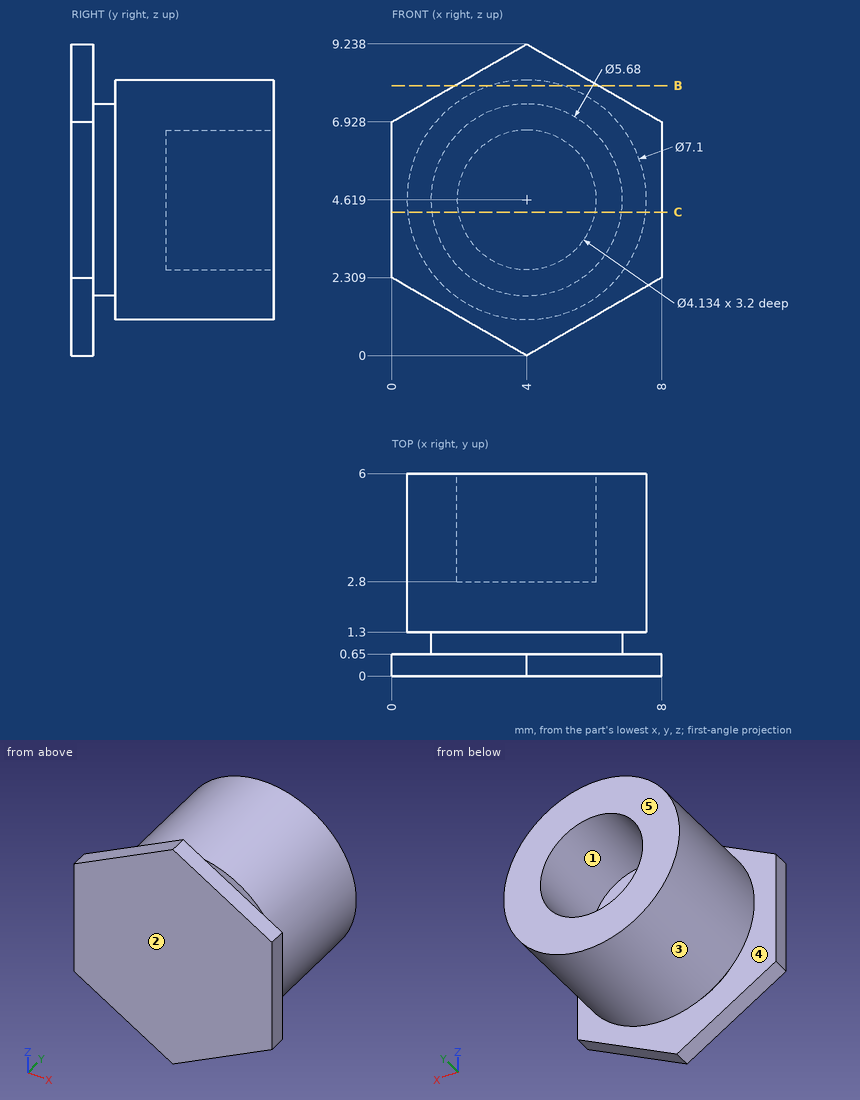
Part print with two shaded views. Sizes in mm from the minimum x, y, z corner. A direction names the side the tool comes from. Coordinates: 2 decimals unless noted, no trailing zeros. Write each loop counter-clockwise with the first axis right and the second up, starting at its lowest first coordinate (ties: lowest second). Pieces come first, ordered by that corner, then holes.
(1) Mould opens along Z. For the marked faces 1, 2 and 3 say: pulls with the +Z half, pulls with the -Z half, needs draft (parallel to the pull), parting line crosses it, or undercut.
(2) Cut at C-C on z = 4.25. List the corners of the cut face in (x, y).
(3) 3-axis set-ups, long thin cutter, end or side, ignore diameter. For the marked faces 4 and 5: which of +Z, -Z, +X, -X, +Y, -Y reach the whole face in a straight line?
(4) Cut at B-B on z = 8. List the corners of the cut face in (x, y).
(5) Pin check, flat tips, straight feed: pin 1 Ø2 at (x, z) = (3.5, 5) entering from +Y; pin 2 Ø3 at (x, y) = (6, 1) entering from +Z (1 decimal). Stop position of each tip, or through.
(6) Drill centre lines: line 1 (Z direction, x = 4, y = 4.1) (1 decimal); line 2 (Y direction, x = 3, z = 6); line 3 (Z direction, x = 2.75, y = 4.25) (1 decimal). Where is each one in solid material? Low to high.
Working result:
1. face 1: undercut
1. face 2: needs draft
1. face 3: parting line crosses it
2. outline: (0, 0) - (8, 0) - (8, 0.65) - (6.82, 0.65) - (6.82, 1.3) - (7.53, 1.3) - (7.53, 6) - (6.03, 6) - (6.03, 2.8) - (1.97, 2.8) - (1.97, 6) - (0.47, 6) - (0.47, 1.3) - (1.18, 1.3) - (1.18, 0.65) - (0, 0.65) - close
3. face 4: none
3. face 5: +Z, -Z, +X, -X, +Y
4. outline: (1.86, 0) - (6.14, 0) - (6.14, 0.65) - (1.86, 0.65) - close; (2.92, 1.3) - (5.08, 1.3) - (5.08, 6) - (2.92, 6) - close
5. pin 1: stops at y = 2.8
5. pin 2: stops at z = 8.9
6. line 1: z = 1.1 to 2.6, 6.7 to 8.2
6. line 2: y = 0 to 2.8
6. line 3: z = 1.3 to 3, 6.3 to 7.9
